Could you check a few things on this model? Use its own coordinates, in mm. Face numbers are marked on the shaded views. A direction names the side the tool comes from. Coordinates: 2 decimals unless noted, no trailing zeros. Order: outer loops, then holes, each group sorted by start corner. A loop starts at its lowest first (then second) coordinate and runs counter-clockwise, first axis right, second up. Notation, with made-up numbers: (-7, -1.5) - (31, -1.5) arc R27 cw to (31, 34.5) - close; hole circle Ø2 at (19.5, 59). An arc over 180 degrees is marked (long way). One line per item, written item: value. Start each with the question number.
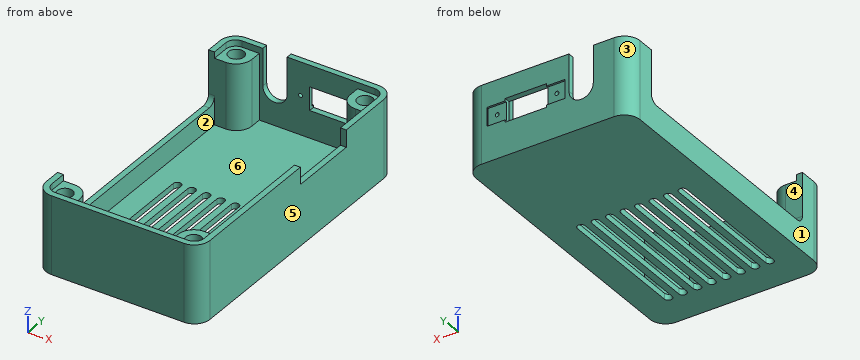
from build123d import *

# Parameters (mm, degrees)
PAD_DEPTH           = 20
SKETCH001_R         = 1.6891
POCKET_DEPTH        = 18.5
POCKET001_DEPTH     = 1.6
POCKET002_DEPTH     = 5
POCKET004_DEPTH     = 5
LINEARPATTERN_COUNT = 8
LINEARPATTERN_PITCH = 3.714286
SKETCH006_W         = 58.2
SKETCH006_H         = 13.0912
POCKET005_DEPTH     = 5
SKETCH009_W         = 20
SKETCH009_H         = 4.8
POCKET007_DEPTH     = 0.5
SKETCH010_R         = 1.98
POCKET011_DEPTH     = 5
SKETCH012_R         = 0.5
POCKET013_DEPTH     = 2
SKETCH013_W         = 10.6
SKETCH013_H         = 6
POCKET014_DEPTH     = 5
SKETCH004_W         = 17.68
SKETCH004_H         = 4.4
POCKET015_DEPTH     = 5
FILLET_R            = 2


with BuildPart() as part:
    # Sketch → Pad (new body)
    with BuildSketch(Plane.XY):
        with BuildLine():
            Line((-17, 37.5), (17, 37.5))
            ThreePointArc((21, 33.5), (19.828427, 36.328427), (17, 37.5))
            Line((21, 33.5), (21, -33.5))
            ThreePointArc((17, -37.5), (19.828427, -36.328427), (21, -33.5))
            Line((17, -37.5), (-17, -37.5))
            ThreePointArc((-21, -33.5), (-19.828427, -36.328427), (-17, -37.5))
            Line((-21, -33.5), (-21, 33.5))
            ThreePointArc((-17, 37.5), (-19.828427, 36.328427), (-21, 33.5))
        make_face()
    extrude(amount=PAD_DEPTH)

    # Sketch001 (on Face10 of Pad) → Pocket (cut)
    with BuildSketch(Plane.XY.offset(20)):
        with Locations((-16.5, -33)):
            Circle(SKETCH001_R)
        with Locations((16.5, -33)):
            Circle(SKETCH001_R)
        with Locations((16.5, 33)):
            Circle(SKETCH001_R)
        with Locations((-16.5, 33)):
            Circle(SKETCH001_R)
        with BuildLine():
            Line((-12.6, 36), (12.6, 36))
            Line((12.6, 36), (12.6, 33.1))
            ThreePointArc((12.6, 33.1), (13.771573, 30.271573), (16.6, 29.1))
            Line((16.6, 29.1), (19.5, 29.1))
            Line((19.5, 29.1), (19.5, -29.1))
            Line((19.5, -29.1), (16.6, -29.1))
            ThreePointArc((16.6, -29.1), (13.771573, -30.271573), (12.6, -33.1))
            Line((12.6, -33.1), (12.6, -36))
            Line((12.6, -36), (-12.6, -36))
            Line((-12.6, -36), (-12.6, -33.1))
            ThreePointArc((-12.6, -33.1), (-13.771573, -30.271573), (-16.6, -29.1))
            Line((-16.6, -29.1), (-19.5, -29.1))
            Line((-19.5, -29.1), (-19.5, 29.1))
            Line((-19.5, 29.1), (-16.6, 29.1))
            ThreePointArc((-16.6, 29.1), (-13.771573, 30.271573), (-12.6, 33.1))
            Line((-12.6, 33.1), (-12.6, 36))
        make_face()
    extrude(amount=-POCKET_DEPTH, mode=Mode.SUBTRACT)

    # Sketch002 (on Face5 of Pocket) → Pocket001 (cut)
    with BuildSketch(Plane.XY.offset(20)):
        with BuildLine():
            Line((-17, 36), (17, 36))
            ThreePointArc((19.5, 33.5), (18.767767, 35.267767), (17, 36))
            Line((19.5, 33.5), (19.5, -33.5))
            ThreePointArc((17, -36), (18.767767, -35.267767), (19.5, -33.5))
            Line((17, -36), (-17, -36))
            ThreePointArc((-19.5, -33.5), (-18.767767, -35.267767), (-17, -36))
            Line((-19.5, -33.5), (-19.5, 33.5))
            ThreePointArc((-17, 36), (-18.767767, 35.267767), (-19.5, 33.5))
        make_face()
    extrude(amount=-POCKET001_DEPTH, mode=Mode.SUBTRACT)

    # Sketch003 (on Face7 of Pocket001) → Pocket002 (cut)
    with BuildSketch(Plane(origin=(0, 37.5, 0), x_dir=(-1, 0, 0), z_dir=(0, 1, 0))):
        with BuildLine():
            Line((5.4685, 10.5), (5.4685, 20))
            Line((5.4685, 20), (11.6915, 20))
            Line((11.6915, 20), (11.6915, 10.5))
            ThreePointArc((5.4685, 10.5), (8.58, 7.3885), (11.6915, 10.5))
        make_face()
    extrude(amount=-POCKET002_DEPTH, mode=Mode.SUBTRACT)

    # Sketch005 → Pocket004 (cut)
    with BuildSketch(Plane(origin=(0, 0, 0), x_dir=(1, 0, 0), z_dir=(0, 0, -1))):
        with BuildLine():
            ThreePointArc((-14, -5), (-13, -6), (-12, -5))
            Line((-12, -5), (-12, 28.5))
            ThreePointArc((-12, 28.5), (-13, 29.5), (-14, 28.5))
            Line((-14, -5), (-14, 28.5))
        make_face()
    pocket004 = extrude(amount=-POCKET004_DEPTH, mode=Mode.SUBTRACT)

    # LinearPattern: Pocket004 ×8
    with Locations(*[(i * LINEARPATTERN_PITCH, 0, 0) for i in range(1, LINEARPATTERN_COUNT)]):
        add(pocket004, mode=Mode.SUBTRACT)

    # Sketch006 (on Face1 of LinearPattern) → Pocket005 (cut)
    with BuildSketch(Plane(origin=(-21, 0, 0), x_dir=(0, -1, 0), z_dir=(-1, 0, 0))):
        with Locations((0, 13.4544)):
            Rectangle(SKETCH006_W, SKETCH006_H)
    extrude(amount=-POCKET005_DEPTH, mode=Mode.SUBTRACT)

    # Sketch009 → Pocket007 (cut)
    with BuildSketch(Plane(origin=(0, 37.5, 0), x_dir=(-1, 0, 0), z_dir=(0, 1, 0))):
        with Locations((-5.6, 11.5088)):
            Rectangle(SKETCH009_W, SKETCH009_H)
    extrude(amount=-POCKET007_DEPTH, mode=Mode.SUBTRACT)

    # Sketch010 → Pocket011 (cut)
    with BuildSketch(Plane.XY.offset(18.4)):
        with Locations((-16.5, 33)):
            Circle(SKETCH010_R)
        with Locations((16.5, 33)):
            Circle(SKETCH010_R)
        with Locations((-16.5, -33)):
            Circle(SKETCH010_R)
        with Locations((16.5, -33)):
            Circle(SKETCH010_R)
    extrude(amount=-POCKET011_DEPTH, mode=Mode.SUBTRACT)

    # Sketch012 → Pocket013 (cut)
    with BuildSketch(Plane(origin=(0, 37, 0), x_dir=(-1, 0, 0), z_dir=(0, 1, 0))):
        with Locations((-13.25, 11.5088)):
            Circle(SKETCH012_R)
        with Locations((2.05, 11.5088)):
            Circle(SKETCH012_R)
    extrude(amount=-POCKET013_DEPTH, mode=Mode.SUBTRACT)

    # Sketch013 (on Face11 of Pocket013) → Pocket014 (cut)
    with BuildSketch(Plane(origin=(0, 37.5, 0), x_dir=(-1, 0, 0), z_dir=(0, 1, 0))):
        with Locations((-5.6, 11.5088)):
            Rectangle(SKETCH013_W, SKETCH013_H)
    extrude(amount=-POCKET014_DEPTH, mode=Mode.SUBTRACT)

    # Sketch004 (on Face14 of Pocket014) → Pocket015 (cut)
    with BuildSketch(Plane.YZ.offset(21)):
        with Locations((10.16, 17.8)):
            Rectangle(SKETCH004_W, SKETCH004_H)
    extrude(amount=-POCKET015_DEPTH, mode=Mode.SUBTRACT)

    # Fillet
    fillet_edges = [part.edges().sort_by_distance(p)[0] for p in [
        (-20.25, 29.1, 6.9088),
        (-20.25, -29.1, 6.9088),
    ]]
    fillet(fillet_edges, radius=FILLET_R)


solid = part.part
Q1. I want a section at A-A on z = 4.25. Please give me the cut outline in (x, y).
Q2. If I drill on L1, parallel to Y at x = -16.5, z = 15.75; L2, parallel to Y at x = -16.5, z = 4.5; L3, parallel to Y at x = 2, z = 2.5, over which ranges is the centre line in solid material (lowest first)?
Q3. I want a section at C-C on y = 21.5. Please give me the cut outline in (x, z), then the cut area to 3 significant figures.
Q4. Which directions (+Z, -Z, +X, -X, +Y, -Y) give clear straight access to the entire face, cutting with the end or side of a thin tool? Please do the marked faces 1 and 2.
Q5. We'd pull the mould along X, two halves only. Please class the marked faces 3, 4, 5 and 6: +X half, -X half, draft (parallel to the pull), parting line (faces both ways), or undercut.
Q6. I'm going to push flat-ended pins straight in: pin 1 (0.8 mm diameter, centred on y = 36.5, z = 11, fed in from +X); pin 2 (3.5 mm diameter, centred on x = -15.5, y = -34, fed in from +Z); pin 3 (12 mm diameter, centred on x = -10, z = 16, fed in from +Y); pin 4 (0.9 mm diameter, centred on y = 35, z = 9.5, fed in from -X). Where does each tip first touch, or does it pass through?
Q7. I want a section at B-B on x = 2. Please give me the cut outline in (y, z).
Q8. I want a section at D-D on y = -25. State how many separate pieces and enclosed holes the cut face has, then the cut area to 3 significant figures.
Values follow:
1. outline: (-21, -33.5) arc R4 ccw to (-17, -37.5) - (17, -37.5) arc R4 ccw to (21, -33.5) - (21, 33.5) arc R4 ccw to (17, 37.5) - (-17, 37.5) arc R4 ccw to (-21, 33.5) - close; hole (-19.5, -29.1) - (-16.6, -29.1) arc R4 cw to (-12.6, -33.1) - (-12.6, -36) - (12.6, -36) - (12.6, -33.1) arc R4 cw to (16.6, -29.1) - (19.5, -29.1) - (19.5, 29.1) - (16.6, 29.1) arc R4 cw to (12.6, 33.1) - (12.6, 36) - (-12.6, 36) - (-12.6, 33.1) arc R4 cw to (-16.6, 29.1) - (-19.5, 29.1) - close; hole circle Ø3.38 at (-16.5, -33); hole circle Ø3.38 at (-16.5, 33); hole circle Ø3.38 at (16.5, -33); hole circle Ø3.38 at (16.5, 33)
2. L1: y = -37.5 to -34.98, -31.02 to -29.1, 29.1 to 31.02, 34.98 to 37.5
2. L2: y = -37.5 to -34.69, -31.31 to -29.1, 29.1 to 31.31, 34.69 to 37.5
2. L3: y = -37.5 to -36, 36 to 37.5
3. outline: (-21, 0) - (21, 0) - (21, 20) - (19.5, 20) - (19.5, 1.5) - (-19.5, 1.5) - (-19.5, 6.91) - (-21, 6.91) - close
3. area: 98.9 mm^2
4. face 1: +Z, -Z, -X, +Y, -Y
4. face 2: +Z
5. face 3: -X half
5. face 4: undercut
5. face 5: +X half
5. face 6: undercut
6. pin 1: stops at x = 20.04
6. pin 2: stops at z = 18.4
6. pin 3: stops at y = 37.5
6. pin 4: stops at x = -20.86
7. outline: (-37.5, 0) - (-29.49, 0) - (-29.49, 1.5) - (-36, 1.5) - (-36, 20) - (-37.5, 20) - close; (5.99, 0) - (37.5, 0) - (37.5, 8.51) - (36, 8.51) - (36, 1.5) - (5.99, 1.5) - close; (36, 14.51) - (37.5, 14.51) - (37.5, 20) - (36, 20) - close
8. separate pieces: 9
8. enclosed holes: 0
8. area: 74.9 mm^2
